```python
from build123d import *

# Parameters (mm, degrees)
SKETCH_1_R          = 12.5
EXTRUDE_1_DEPTH     = 2
SKETCH_2_R          = 7.5
EXTRUDE_2_DEPTH     = 3
FILLET_1_R          = 1
CUT_EXTRUDE_1_REACH = 20.371
SKETCH_3_R          = 3


with BuildPart() as part:
    # 草图1 → 凸台-拉伸1 (new body)
    with BuildSketch(Plane(origin=(0, 0, 0), x_dir=(1, 0, 0), z_dir=(0, 1, 0))):
        with Locations(Location((0, 0, 0), (0, 0, 270))):
            Circle(SKETCH_1_R)
    extrude(amount=EXTRUDE_1_DEPTH)

    # 草图2 → 凸台-拉伸2 (add)
    with BuildSketch(Plane(origin=(0, 2, 0), x_dir=(1, 0, 0), z_dir=(0, 1, 0))):
        with Locations(Location((0, 0, 0), (0, 0, 270))):
            Circle(SKETCH_2_R)
    extrude(amount=EXTRUDE_2_DEPTH)

    # 圆角1
    fillet_1_edges = [part.edges().sort_by_distance(p)[0] for p in [
        (0, 2, -7.5),
    ]]
    fillet(fillet_1_edges, radius=FILLET_1_R)

    # 草图3 → 切除-拉伸1 (cut, up to next)
    with BuildSketch(Plane(origin=(0, 5, 0), x_dir=(1, 0, 0), z_dir=(0, 1, 0)), mode=Mode.PRIVATE) as cut_extrude_1_sk1:
        with Locations(Location((0, 0, 0), (0, 0, 270))):
            Circle(SKETCH_3_R)
    cut_extrude_1_tool1 = extrude(cut_extrude_1_sk1.sketch, amount=-CUT_EXTRUDE_1_REACH, mode=Mode.PRIVATE) & part.part
    add(cut_extrude_1_tool1.solids().sort_by_distance((0, 5, 0))[0], mode=Mode.SUBTRACT)


solid = part.part
```
Could you check a few things on this model? Use its own coordinates, in mm. A direction names the side the tool comes from. Round coordinates to 2 decimals unless told otherwise and drop trailing zeros. Order: outer loops, then holes, each group sorted by start corner. A loop starts at its lowest first (then second) coordinate and runs counter-clockwise, first axis right, second up. Notation, with made-up numbers: M -24,-36.5 L -12,-36.5 A6 ccw -12,-29.5 Z; hole C -38.75,-32 d10. An arc over 180 degrees is marked long. One line per question, with ' | ' between items. Start each with the question number.
(1) Please list where these lines run through material, in increasing order: line 1 along X through (y, z) = (3.95, 0); line 2 along Y through (x, z) = (-11, -2); line 3 along X through (y, z) = (2.1, -1.25).
(2) Suppose I cut it at C-C on y = 4.4. List the corners of the cut face in (x, z) for me, then the cut area to 3 significant figures.
(3) For P1, Ø2, axis at y = 1, z = -1.5, coming from the +X side, with a flat end and sliding along its axis, tell me the tip position at first contact or that it passes through.
(4) For faces 1 (the face through (0.1, 5, 3.2)), 2 (the face through (0.33, 3.986, -7.493)), which set-ups out of +Z, -Z, +X, -X, +Y, -Y let a thin tool reach every point of the face, with its end or its side?
(5) Suppose I cut it at B-B on x = 0. List the corners of the cut face in (y, z) for me, then the cut area to 3 significant figures.
(6) Suppose I cut it at A-A on z = 0. List the corners of the cut face in (x, y) for me, then the cut area to 3 significant figures.
(7) Suppose I cut it at D-D on x = -11. List the corners of the cut face in (y, z) for me.
(8) Thinking about a two-plate mould opening in X: for faces 3 (the face through (0.9, 2.54, 2.86)), 4 (the face through (3, 2, 8.2)), 5 (the face through (3.755, 0.986, 11.923)), which applies, +X half, -X half, draft (parallel to the pull), parting line (faces both ways), or undercut?
Geometry results:
1) line 1: -7.5 to -3, 3 to 7.5 | line 2: 0 to 2 | line 3: -7.97 to -2.73, 2.73 to 7.97
2) outline: C 0,0 d15; hole C 0,0 d6 | area: 148 mm²
3) P1: x = 12.49
4) face 1: +Z, -Z, +X, -X, +Y | face 2: +Y
5) outline: M 0,-12.5 L 2,-12.5 L 2,-8.5 A1 cw 3,-7.5 L 5,-7.5 L 5,-3 L 0,-3 Z; M 0,3 L 5,3 L 5,7.5 L 3,7.5 A1 cw 2,8.5 L 2,12.5 L 0,12.5 Z | area: 65.4 mm²
6) outline: M -12.5,0 L -3,0 L -3,5 L -7.5,5 L -7.5,3 A1 cw -8.5,2 L -12.5,2 Z; M 3,0 L 12.5,0 L 12.5,2 L 8.5,2 A1 cw 7.5,3 L 7.5,5 L 3,5 Z | area: 65.4 mm²
7) outline: M 0,-5.94 L 2,-5.94 L 2,5.94 L 0,5.94 Z
8) face 3: undercut | face 4: draft | face 5: parting line
